Source: CAD feature listing. Evaluate the final solid. Frame: model axes, mm. Face numbers are marked on the shaded views. A direction names the side the tool comes from. Give positions to 0.01 mm unless a question says otherwise; leave off trailing zeros. Loops run counter-clockwise (first coordinate to the right, second up) from the corner with the lowest first, then second, coordinate; pieces in that order, holes last. Notation, with made-up numbers: (-34, -24.5) - (0, -24.5) arc R12 cw to (0, -15.5) - close; hole circle Ø10 at (-6, 67). An arc over 180 degrees is marked (long way). Put each result on its own line as item: value.
```python
from build123d import *

# Parameters (mm, degrees)
SKETCH_W        = 70
SKETCH_H        = 70
PAD_DEPTH       = 2
PAD001_DEPTH    = 22
POCKET_DEPTH    = 22
SKETCH003_W     = 16
SKETCH003_H     = 23.864653
POCKET001_DEPTH = 18
SKETCH009_R     = 1.6
POCKET005_DEPTH = 58.501
SKETCH010_R     = 2
SKETCH010_W     = 2.5
SKETCH010_H     = 3
SKETCH010_W_2   = 3
PAD004_DEPTH    = 7
POCKET006_DEPTH = 5
POCKET007_DEPTH = 2
FILLET_R        = 15
SKETCH014_W     = 3
SKETCH014_H     = 4
POCKET009_DEPTH = 4
SKETCH015_R     = 1
POCKET010_DEPTH = 24.001
SKETCH016_R     = 1
SKETCH016_W     = 37
SKETCH016_H     = 37
POCKET011_DEPTH = 5


with BuildPart() as part:
    # Sketch → Pad (new body)
    with BuildSketch(Plane.XY):
        Rectangle(SKETCH_W, SKETCH_H)
        with BuildLine():
            ThreePointArc((27.608372, -4.666667), (28, 0), (27.608372, 4.666667))
            ThreePointArc((31.552426, 5.333333), (29.247066, 6.972027), (27.608372, 4.666667))
            ThreePointArc((31.552426, -5.333333), (32, 0), (31.552426, 5.333333))
            ThreePointArc((27.608372, -4.666667), (29.247066, -6.972027), (31.552426, -5.333333))
        make_face(mode=Mode.SUBTRACT)
        with BuildLine():
            ThreePointArc((-27.608372, 4.666667), (-28, 0), (-27.608372, -4.666667))
            ThreePointArc((-31.552426, -5.333333), (-29.247066, -6.972027), (-27.608372, -4.666667))
            ThreePointArc((-31.552426, 5.333333), (-32, 0), (-31.552426, -5.333333))
            ThreePointArc((-27.608372, 4.666667), (-29.247066, 6.972027), (-31.552426, 5.333333))
        make_face(mode=Mode.SUBTRACT)
        with BuildLine():
            ThreePointArc((4.666667, 27.608372), (-1e-06, 28), (-4.666668, 27.608372))
            ThreePointArc((-5.333333, 31.552426), (-6.972027, 29.247066), (-4.666668, 27.608372))
            ThreePointArc((5.333333, 31.552426), (0, 32), (-5.333333, 31.552426))
            ThreePointArc((4.666667, 27.608372), (6.972027, 29.247066), (5.333333, 31.552426))
        make_face(mode=Mode.SUBTRACT)
        with BuildLine():
            ThreePointArc((-4.666659, -27.608374), (4e-06, -28), (4.666667, -27.608372))
            ThreePointArc((5.333333, -31.552426), (6.972027, -29.247066), (4.666667, -27.608372))
            ThreePointArc((-5.333319, -31.552428), (7e-06, -32), (5.333333, -31.552426))
            ThreePointArc((-4.666659, -27.608374), (-6.972027, -29.247069), (-5.333319, -31.552428))
        make_face(mode=Mode.SUBTRACT)
    extrude(amount=PAD_DEPTH)

    # Sketch001 (on Face22 of Pad) → Pad001 (join)
    with BuildSketch(Plane.XY.offset(2)):
        with BuildLine():
            Line((21.719807, -23.5), (-21.719807, -23.5))
            ThreePointArc((-23.5, -21.719807), (-22.627417, -22.627417), (-21.719807, -23.5))
            Line((-23.5, 21.719807), (-23.5, -21.719807))
            ThreePointArc((-21.719807, 23.5), (-22.627417, 22.627417), (-23.5, 21.719807))
            Line((-21.719807, 23.5), (21.719807, 23.5))
            ThreePointArc((23.5, 21.719807), (22.627417, 22.627417), (21.719807, 23.5))
            Line((23.5, 21.719807), (23.5, -21.719807))
            ThreePointArc((21.719807, -23.5), (22.627417, -22.627417), (23.5, -21.719807))
        make_face()
    extrude(amount=PAD001_DEPTH)

    # Sketch002 (on Face31 of Pad001) → Pocket (cut)
    with BuildSketch(Plane.XY.offset(24)):
        with BuildLine():
            Line((-22.3, 21.244999), (-22.3, -21.244999))
            ThreePointArc((-22.3, -21.244999), (-21.778889, -21.778889), (-21.244999, -22.3))
            Line((-21.244999, -22.3), (21.244999, -22.3))
            ThreePointArc((21.244999, -22.3), (21.778889, -21.778889), (22.3, -21.244999))
            Line((22.3, 21.244999), (22.3, -21.244999))
            ThreePointArc((22.3, 21.244999), (21.778889, 21.778889), (21.244999, 22.3))
            Line((-21.244999, 22.3), (21.244999, 22.3))
            ThreePointArc((-21.244999, 22.3), (-21.778889, 21.778889), (-22.3, 21.244999))
        make_face()
    extrude(amount=-POCKET_DEPTH, mode=Mode.SUBTRACT)

    # Sketch003 (on Face30 of Pocket) → Pocket001 (cut)
    with BuildSketch(Plane.XZ.offset(23.5)):
        with Locations((12.5, 21.932326)):
            Rectangle(SKETCH003_W, SKETCH003_H)
    extrude(amount=-POCKET001_DEPTH, mode=Mode.SUBTRACT)

    # Sketch009 → Pocket005 (cut, through all)
    with BuildSketch(Plane.XZ.offset(23.5)):
        with Locations((0, 20)):
            Circle(SKETCH009_R)
    extrude(amount=-POCKET005_DEPTH, mode=Mode.SUBTRACT)

    # Sketch010 (on Face45 of Pocket005) → Pad004 (join)
    with BuildSketch(Plane.XY.offset(2)):
        with Locations((21, 21)):
            Circle(SKETCH010_R)
        with Locations((-21, 21)):
            Circle(SKETCH010_R)
        with Locations((-21, -21)):
            Circle(SKETCH010_R)
        with Locations((21.75, 4.5)):
            Rectangle(SKETCH010_W, SKETCH010_H)
        with Locations((0, -21)):
            Rectangle(SKETCH010_W_2, SKETCH010_H)
    extrude(amount=PAD004_DEPTH)

    # Sketch011 (on Face26 of Pad004) → Pocket006 (cut)
    with BuildSketch(Plane(origin=(0, 23.5, 0), x_dir=(-1, 0, 0), z_dir=(0, 1, 0))):
        with BuildLine():
            Line((-18.5, 17.993099), (-18.5, 5.993099))
            ThreePointArc((-18.5, 5.993099), (-16.5, 3.993099), (-14.5, 5.993099))
            Line((-14.5, 17.993099), (-14.5, 5.993099))
            ThreePointArc((-14.5, 17.993099), (-16.5, 19.993099), (-18.5, 17.993099))
        make_face()
        with BuildLine():
            Line((-7.5, 17.993099), (-7.5, 5.993099))
            ThreePointArc((-7.5, 5.993099), (-5.5, 3.993099), (-3.5, 5.993099))
            Line((-3.5, 17.993099), (-3.5, 5.993099))
            ThreePointArc((-3.5, 17.993099), (-5.5, 19.993099), (-7.5, 17.993099))
        make_face()
        with BuildLine():
            Line((3.5, 17.993099), (3.5, 5.993099))
            ThreePointArc((3.5, 5.993099), (5.5, 3.993099), (7.5, 5.993099))
            Line((7.5, 17.993099), (7.5, 5.993099))
            ThreePointArc((7.5, 17.993099), (5.5, 19.993099), (3.5, 17.993099))
        make_face()
        with BuildLine():
            Line((14.5, 17.993099), (14.5, 5.993099))
            ThreePointArc((14.5, 5.993099), (16.5, 3.993099), (18.5, 5.993099))
            Line((18.5, 17.993099), (18.5, 5.993099))
            ThreePointArc((18.5, 17.993099), (16.5, 19.993099), (14.5, 17.993099))
        make_face()
    extrude(amount=-POCKET006_DEPTH, mode=Mode.SUBTRACT)

    # Sketch012 (on Face30 of Pocket006) → Pocket007 (cut)
    with BuildSketch(Plane.XZ.offset(23.5)):
        with BuildLine():
            Line((-17, 18), (-17, 6))
            ThreePointArc((-17, 6), (-15, 4), (-13, 6))
            Line((-13, 18), (-13, 6))
            ThreePointArc((-13, 18), (-15, 20), (-17, 18))
        make_face()
        with BuildLine():
            Line((-6, 18), (-6, 6))
            ThreePointArc((-6, 6), (-4, 4), (-2, 6))
            Line((-2, 18), (-2, 6))
            ThreePointArc((-2, 18), (-4, 20), (-6, 18))
        make_face()
    extrude(amount=-POCKET007_DEPTH, mode=Mode.SUBTRACT)

    # Fillet
    fillet_edges = [part.edges().sort_by_distance(p)[0] for p in [
        (-35, -35, 1),
        (-35, 35, 1),
        (35, -35, 1),
        (35, 35, 1),
    ]]
    fillet(fillet_edges, radius=FILLET_R)

    # Sketch014 (on Face2 of Fillet) → Pocket009 (cut)
    with BuildSketch(Plane(origin=(0, 0, 0), x_dir=(1, 0, 0), z_dir=(0, 0, -1))):
        with Locations((-23.5, -11)):
            Rectangle(SKETCH014_W, SKETCH014_H)
    extrude(amount=-POCKET009_DEPTH, mode=Mode.SUBTRACT)

    # Sketch015 (on Face2 of Pocket009) → Pocket010 (cut, through all)
    with BuildSketch(Plane(origin=(0, 0, 0), x_dir=(1, 0, 0), z_dir=(0, 0, -1))):
        with Locations((-21, 21)):
            Circle(SKETCH015_R)
        with Locations((-21, -21)):
            Circle(SKETCH015_R)
    extrude(amount=-POCKET010_DEPTH, mode=Mode.SUBTRACT)

    # Sketch016 (on Face44 of Pocket010) → Pocket011 (cut)
    with BuildSketch(Plane(origin=(0, 0, 4), x_dir=(1, 0, 0), z_dir=(0, 0, -1))):
        with Locations((15.5, 25.5)):
            Circle(SKETCH016_R)
        with Locations((-15.5, 25.5)):
            Circle(SKETCH016_R)
        with Locations((-15.5, -25.5)):
            Circle(SKETCH016_R)
        with Locations((15.5, -25.5)):
            Circle(SKETCH016_R)
        Rectangle(SKETCH016_W, SKETCH016_H)
    extrude(amount=POCKET011_DEPTH, mode=Mode.SUBTRACT)


solid = part.part
```
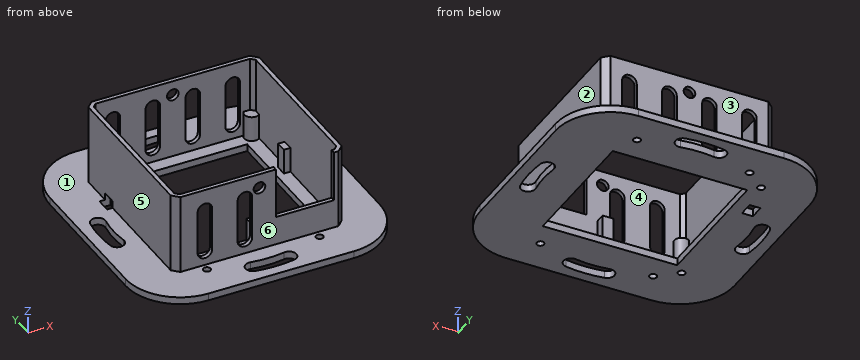
1) Mould query, pull axis X, two halves, no side actions, for the marked faces 4, 5 and 6. Classes: pulls with the +X half, pulls with the -X half, needs draft (parallel to the pull), parting line crosses it, or undercut.
Check result:
face 4: undercut
face 5: pulls with the -X half
face 6: needs draft
2) Material intervals for line 1 along Y through (x, z) = (-15.5, 1.15); line 2 along X through (y, z) = (21, 3.5); line 3 along X through (y, z) = (10, 13.75), sorted ascending. Write a range as [from, to].
Check result:
line 1: [-35, -26.5], [-24.5, -18.5], [18.5, 24.5], [26.5, 35]
line 2: [-23.5, -22], [-20, -19], [19, 23.5]
line 3: [-23.5, -22.3], [22.3, 23.5]
3) Section query B-B, the plane x = 0. State how many separate pieces and enclosed holes the cut face has, plus the area to 3 significant figures.
Check result:
separate pieces: 6
enclosed holes: 0
area: 115 mm²
4) Section query A-A, the plane y = -11.5. Output: boundary loops of the cut face in (x, z), plus the area to 3 significant figures.
Check result:
outline: (-35, 0) - (-18.5, 0) - (-18.5, 2) - (-22.3, 2) - (-22.3, 24) - (-23.5, 24) - (-23.5, 2) - (-35, 2) - close; (18.5, 0) - (35, 0) - (35, 2) - (23.5, 2) - (23.5, 24) - (22.3, 24) - (22.3, 2) - (18.5, 2) - close
area: 119 mm²
5) Pin query (flat end, axial travel): P1, Ø1.4, axis at x = 21.5, y = 5, coming from the +Z side; P2, Ø1.8, axis at x = 15.5, y = 25.5, coming from the +Z side; P3, Ø10, axis at y = 9, z = 9, coming from the +X side; P4, Ø3, axis at x = 24.5, z = 18.5, coming from the -Y side. Return the tip coordinate at first contact, or that it passes through.
Check result:
P1: z = 9
P2: through
P3: x = 23.5
P4: y = -22.25
6) Access query for the marked faces 1, 2 and 3. Directions: +Z, -Z, +X, -X, +Y, -Y. A direction counts if a zero-diameter tool reaches every point of the face in a straight line with its end or side. Return the directions, or none.
Check result:
face 1: +Z
face 2: +Z, +X, +Y, -Y
face 3: +Z, +X, -X, +Y
